from build123d import *

# Parameters (mm, degrees)
BOSS_EXTRUDE1_DEPTH     = 25.4
SKETCH2_R               = 6.35
CUT_EXTRUDE1_DEPTH      = 56.660932074
CUT_EXTRUDE2_DEPTH      = 53.31230942
CUT_EXTRUDE2_DEPTH_BACK = 53.31230942
SKETCH5_R               = 3.302


with BuildPart() as part:
    # Sketch1 → Boss-Extrude1 (new body)
    with BuildSketch(Plane(origin=(0, 0, 0), x_dir=(1, 0, 0), z_dir=(0, 1, 0))):
        Polygon((0, 0), (0, 38.1), (6.35, 38.1), (6.35, 6.35), (25.294420667, 6.35), (25.294420667, 38.1), (31.644420667, 38.1), (31.644420667, 0), align=None)
    extrude(amount=BOSS_EXTRUDE1_DEPTH)

    # Sketch2 → Cut-Extrude1 (cut, through all)
    with BuildSketch(Plane.XY):
        with Locations((15.822210333, 12.7)):
            Circle(SKETCH2_R)
    extrude(amount=-CUT_EXTRUDE1_DEPTH, mode=Mode.SUBTRACT)

    # Sketch5 → Cut-Extrude2 (cut, two sides: drawn at the far end of the back side and taken through both)
    with BuildSketch(Plane(origin=(6.35, 0, 0), x_dir=(0, 0, -1), z_dir=(1, 0, 0)).offset(-CUT_EXTRUDE2_DEPTH_BACK)):
        with Locations((22.86, 12.7)):
            Circle(SKETCH5_R)
    extrude(amount=CUT_EXTRUDE2_DEPTH + CUT_EXTRUDE2_DEPTH_BACK, mode=Mode.SUBTRACT)


solid = part.part
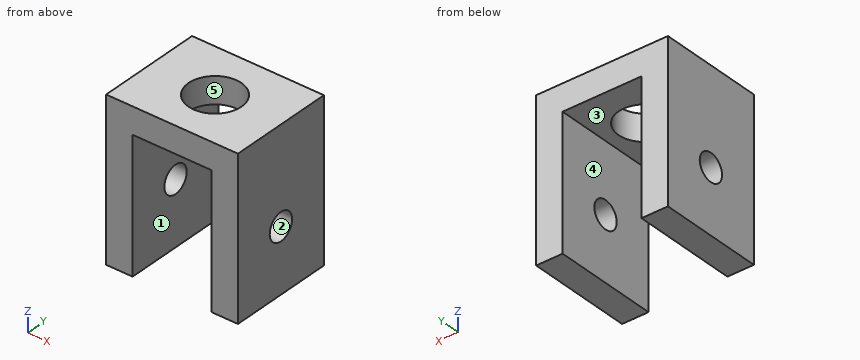
Here's how the part is built. I have some questions about the finished solid (model axes, mm). Face numbers are marked on the shaded views. A direction names the side the tool comes from. Round coordinates to 2 decimals unless told otherwise and drop trailing zeros. Loops run counter-clockwise (first coordinate to the right, second up) from the corner with the lowest first, then second, coordinate; pieces in that order, holes last. Notation, with made-up numbers: (63.25, 76) -> (92.25, 76) arc R11 cw to (92.25, 80) -> close; hole circle Ø4 at (67.25, 54). An arc over 180 degrees is marked (long way). Write each question's results on one line, items separated by ' | '.
(1) We'd pull the mould along Z, two halves only. Please class the marked faces 1, 2 and 3: released by +Z, released by -Z, zero draft, split by the parting line, or undercut.
Worked answers:
face 1: zero draft | face 2: undercut | face 3: released by -Z
(2) For P1, Ø5.5, axis at x = 11.5, y = 11, coming from the -Z side, with a flat end and sliding along its axis, tell me the tip position at first contact or that it passes through.
Worked answers:
P1: z = -6.35
(3) If we section it at C-C, the plane x = 30: List the corners of the cut face in (y, z) for me.
Worked answers:
outline: (0, -38.1) -> (25.4, -38.1) -> (25.4, 0) -> (0, 0) -> close; hole circle Ø6.6 at (12.7, -22.86)
(4) If we section it at A-A, the plane y = 12.7: List the corners of the cut face in (x, z) for me, then the cut area to 3 significant figures.
Worked answers:
outline: (0, -38.1) -> (6.35, -38.1) -> (6.35, -26.16) -> (0, -26.16) -> close; (0, -19.56) -> (6.35, -19.56) -> (6.35, -6.35) -> (9.47, -6.35) -> (9.47, 0) -> (0, 0) -> close; (22.17, -6.35) -> (25.29, -6.35) -> (25.29, -19.56) -> (31.64, -19.56) -> (31.64, 0) -> (22.17, 0) -> close; (25.29, -38.1) -> (31.64, -38.1) -> (31.64, -26.16) -> (25.29, -26.16) -> close | area: 440 mm2
(5) For the marked faces 4 and 5, which set-ups out of +Z, -Z, +X, -X, +Y, -Y let a thin tool reach every point of the face, with its end or its side?
Worked answers:
face 4: -Z, +Y, -Y | face 5: +Z, -Z
(6) If we section it at D-D, the plane y = 8.25: List the corners of the cut face in (x, z) for me.
Worked answers:
outline: (0, -38.1) -> (6.35, -38.1) -> (6.35, -6.35) -> (11.29, -6.35) -> (11.29, 0) -> (0, 0) -> close; (20.35, -6.35) -> (25.29, -6.35) -> (25.29, -38.1) -> (31.64, -38.1) -> (31.64, 0) -> (20.35, 0) -> close
(7) If we section it at B-B, the plane z = -22.86: List the corners of the cut face in (x, y) for me.
Worked answers:
outline: (0, 0) -> (6.35, 0) -> (6.35, 9.4) -> (0, 9.4) -> close; (0, 16) -> (6.35, 16) -> (6.35, 25.4) -> (0, 25.4) -> close; (25.29, 0) -> (31.64, 0) -> (31.64, 9.4) -> (25.29, 9.4) -> close; (25.29, 16) -> (31.64, 16) -> (31.64, 25.4) -> (25.29, 25.4) -> close
(8) If I drill on L1, parallel to X at y = 16.5, z = -9.5; L2, parallel to Z at x = 28.5, y = 12.7; L3, parallel to Z at x = 17.5, y = 21.75, over which ranges is the centre line in solid material (lowest first)?
Worked answers:
L1: 0 to 6.35, 25.29 to 31.64 | L2: -38.1 to -26.16, -19.56 to 0 | L3: -6.35 to 0
